Build history of the part. All positions in model axes, mm. A direction names the side the tool comes from. Give positions to 0.01 mm unless a question says otherwise; leave off trailing zeros. Order: outer loops, then holes, each group sorted by start corner. A loop starts at its lowest first (then second) coordinate and runs counter-clockwise, first axis right, second up. Notation, with made-up numbers: (56, -25.5) - (103, -25.5) arc R29 cw to (103, 11.5) - close; hole circle Ø1 at (75, 45.25). An arc over 180 degrees is marked (long way). Answer in a Markdown table with one row per item.
```python
from build123d import *

# Parameters (mm, degrees)
F0_R     = 1.5
F0_R_2   = 2
F0_W     = 30
F0_H     = 30
F1_DEPTH = 3


# Not quite as in the source:
# - ends of sketch curves that miss each other by under 0.0002 mm in the source are joined


with BuildPart() as f1:
    # F0 (on Front) → F1 (new body)
    with BuildSketch(Plane.XZ):
        with BuildLine():
            Line((27.5, 17.5), (27.5, 27.5))
            Line((27.5, 27.5), (17.5, 27.5))
            add(Edge.make_bspline(
                [(17.5, 27.5), (0, 19.2440692335), (0, 19.2440692335), (-17.5, 27.5)],
                knots=[0, 0, 0, 0, 35, 35, 35, 35], degree=3))
            Line((-17.5, 27.5), (-27.5, 27.5))
            Line((-27.5, 27.5), (-27.5, 17.5))
            add(Edge.make_bspline(
                [(-27.5, 17.5), (-19.2440692335, 0), (-19.2440692335, 0), (-27.5, -17.5)],
                knots=[0, 0, 0, 0, 35, 35, 35, 35], degree=3))
            Line((-27.5, -17.5), (-27.5, -27.5))
            Line((-27.5, -27.5), (-17.5, -27.5))
            add(Edge.make_bspline(
                [(-17.5, -27.5), (0, -19.2440692335), (0, -19.2440692335), (17.5, -27.5)],
                knots=[0, 0, 0, 0, 35, 35, 35, 35], degree=3))
            Line((17.5, -27.5), (27.5, -27.5))
            Line((27.5, -27.5), (27.5, -17.5))
            add(Edge.make_bspline(
                [(27.5, -17.5), (19.2440690845, 0), (19.2440692335, 0), (27.5, 17.5)],
                knots=[0, 0, 0, 0, 35, 35, 35, 35], degree=3))
        make_face()
        with Locations((-22.9809703886, -22.9809703886)):
            Circle(F0_R, mode=Mode.SUBTRACT)
        with Locations((-18.7383297014, -18.7383297014)):
            Circle(F0_R_2, mode=Mode.SUBTRACT)
        with Locations((22.9809703886, -22.9809703886)):
            Circle(F0_R, mode=Mode.SUBTRACT)
        with Locations((18.7383297014, -18.7383297014)):
            Circle(F0_R_2, mode=Mode.SUBTRACT)
        with Locations((-18.7383297014, 18.7383297014)):
            Circle(F0_R_2, mode=Mode.SUBTRACT)
        with Locations((-22.9809703886, 22.9809703886)):
            Circle(F0_R, mode=Mode.SUBTRACT)
        Rectangle(F0_W, F0_H, mode=Mode.SUBTRACT)
        with Locations((18.7383297014, 18.7383297014)):
            Circle(F0_R_2, mode=Mode.SUBTRACT)
        with Locations((22.9809703886, 22.9809703886)):
            Circle(F0_R, mode=Mode.SUBTRACT)
    extrude(amount=F1_DEPTH)


solid = f1.part
```
1. Cut at A-A on x = -20. Write the cut outline in (y, z), and give its area (3 significant figures).
Check result:
| item | result |
|---|---|
| outline | (-3, -27.5) - (0, -27.5) - (0, -20.29) - (-3, -20.29) - close; (-3, -17.19) - (0, -17.19) - (0, 17.19) - (-3, 17.19) - close; (-3, 20.29) - (0, 20.29) - (0, 27.5) - (-3, 27.5) - close |
| area | 146 mm² |
2. Two-plate mould, pull along X, no slides. Class faces 1 (the face through (0, -1, 15)), 2 (the face through (22, -1, -27.5)), 3 (the face through (27.5, -1, -23)): +X half, -X half, draft (parallel to the pull), parting line (faces both ways), or undercut.
Check result:
| item | result |
|---|---|
| face 1 | undercut |
| face 2 | draft |
| face 3 | +X half |
3. Drop flat-ended pins along their axis: P1, Ø3.5, axis at x = -18.74, z = -18.74, coming from the -Y side; P2, Ø0.9, axis at x = 7.5, y = -1, coming from the -Z side; P3, Ø1.5, axis at y = -1, z = -0.5, coming from the +X side. Give the stop position or say it passes through.
Check result:
| item | result |
|---|---|
| P1 | passes through |
| P2 | stops at z = -23.18 |
| P3 | stops at x = 21.36 |
4. Cut at B-B on x = 23. Count the separate pieces of the cut face and the enclosed holes in it, and give its area (3 significant figures).
Check result:
| item | result |
|---|---|
| separate pieces | 4 |
| enclosed holes | 0 |
| area | 102 mm² |
5. Probe line 1 (X direction, y = -1, z = 0.5); line 2 (Z direction, x = -17, y = -1.55); line 3 (Z direction, x = -24, y = -2.75). List the from-to ranges inside material, lowest first.
Check result:
| item | result |
|---|---|
| line 1 | x = -21.32 to -15, 15 to 21.32 |
| line 2 | z = -27.26 to -19.73, -17.75 to 17.75, 19.73 to 27.26 |
| line 3 | z = -27.5 to -24.08, -21.88 to -9.91, 9.91 to 21.88, 24.08 to 27.5 |
6. Which spindle directions (+Z, -Z, +X, -X, +Y, -Y) get a long thin tool onto all of the face, cutting with end or side? Do faces 4 (the face through (0, -3, 19)), 5 (the face through (0, -1, -15)). Say none if no direction does.
Check result:
| item | result |
|---|---|
| face 4 | +Z, -Z, +X, -X, -Y |
| face 5 | +Y, -Y |
